Source: CAD feature listing. Evaluate the final solid. Frame: model axes, mm. A direction names the side the tool comes from. Give positions to 0.01 mm unless a question says otherwise; leave off trailing zeros. Loops run counter-clockwise (first coordinate to the right, second up) from the corner with the lowest first, then second, coordinate; pieces in that order, holes last. Notation, with made-up numbers: M -12.75,57 L 0.25,57 A31 cw 0.25,86 Z; hole C 6.25,4.25 d6. An arc over 180 degrees is marked long. Put each result on its own line as item: value.
from build123d import *

# Parameters (mm, degrees)
SKETCH1_W           = 80
SKETCH1_H           = 80
BOSS_EXTRUDE1_DEPTH = 4
CUT_EXTRUDE2_REACH  = 58.71
SKETCH3_R           = 1.75
SKETCH4_W           = 80
SKETCH4_H           = 80
CUT_EXTRUDE3_DEPTH  = 4
SKETCH2_R           = 2.95
BOSS_EXTRUDE2_DEPTH = 8


with BuildPart() as part:
    # Sketch1 → Boss-Extrude1 (new body)
    with BuildSketch(Plane(origin=(0, 0, 0), x_dir=(1, 0, 0), z_dir=(0, 1, 0))):
        Rectangle(SKETCH1_W, SKETCH1_H)
    extrude(amount=BOSS_EXTRUDE1_DEPTH)

    # Sketch3 → Cut-Extrude2 (cut, up to next)
    with BuildSketch(Plane(origin=(0, 4, 0), x_dir=(1, 0, 0), z_dir=(0, 1, 0)), mode=Mode.PRIVATE) as cut_extrude2_sk1:
        with Locations(Location((20.666851305, 33.07387575, 0), (0, 0, 270))):
            Circle(SKETCH3_R)
    cut_extrude2_tool1 = extrude(cut_extrude2_sk1.sketch, amount=-CUT_EXTRUDE2_REACH, mode=Mode.PRIVATE) & part.part
    # Sketch3 → Cut-Extrude2 (cut, up to next)
    with BuildSketch(Plane(origin=(0, 4, 0), x_dir=(1, 0, 0), z_dir=(0, 1, 0)), mode=Mode.PRIVATE) as cut_extrude2_sk2:
        with Locations(Location((-20.666851305, 33.07387575, 0), (0, 0, 90))):
            Circle(SKETCH3_R)
    cut_extrude2_tool2 = extrude(cut_extrude2_sk2.sketch, amount=-CUT_EXTRUDE2_REACH, mode=Mode.PRIVATE) & part.part
    add(cut_extrude2_tool1.solids().sort_by_distance((20.666851, 4, -33.073876))[0], mode=Mode.SUBTRACT)
    add(cut_extrude2_tool2.solids().sort_by_distance((-20.666851, 4, -33.073876))[0], mode=Mode.SUBTRACT)

    # Sketch4 → Cut-Extrude3 (cut)
    with BuildSketch(Plane(origin=(0, 4, 0), x_dir=(1, 0, 0), z_dir=(0, 1, 0))):
        Rectangle(SKETCH4_W, SKETCH4_H)
        Polygon((5, 8), (18.946402637, 37.908156972), (25.290557147, 34.94982914), (6.195338219, -6), (0, -6), (-6.195338219, -6), (-25.290557147, 34.94982914), (-18.946402637, 37.908156972), (-5, 8), (0, 8), align=None, mode=Mode.SUBTRACT)
    extrude(amount=-CUT_EXTRUDE3_DEPTH, mode=Mode.SUBTRACT)

    # Sketch2 → Boss-Extrude2 (add)
    with BuildSketch(Plane(origin=(0, 4, 0), x_dir=(1, 0, 0), z_dir=(0, 1, 0))):
        with Locations(Location((0, 0, 0), (0, 0, 270))):
            Circle(SKETCH2_R)
    extrude(amount=BOSS_EXTRUDE2_DEPTH)


solid = part.part
1. Section query A-A (x = 0). Output: boundary loops of the cut face in (y, z), plus the area to 3 significant figures.
Found:
outline: M 0,-8 L 4,-8 L 4,-2.95 L 12,-2.95 L 12,2.95 L 4,2.95 L 4,6 L 0,6 Z
area: 103 mm^2
2. Draft query along Z for faces 4 (the cylindrical face through (-20.744, 2.028, -31.326)), 5 (the flat face through (11.876, 2.028, -22.745)), 6 (the flat face through (0, 12, 0)). Return one class per face: pulls with the +Z half, pulls with the -Z half, needs draft (parallel to the pull), parting line crosses it, or undercut.
Found:
face 4: undercut
face 5: pulls with the -Z half
face 6: needs draft
3. Material intervals for line 1 (Y direction, x = 5, z = 3.5); line 2 (X direction, y = 3.25, z = -25); line 3 (Z direction, x = 19.5, y = 1.75), sorted ascending. Write a range as from..to.
Found:
line 1: 0..4
line 2: -20.65..-12.93, 12.93..20.65
line 3: -37.65..-34.38, -31.77..-22.53
4. Section query C-C (z = -14). Output: boundary loops of the cut face in (x, y).
Found:
outline: M -15.52,0 L -7.8,0 L -7.8,4 L -15.52,4 Z; M 7.8,0 L 15.52,0 L 15.52,4 L 7.8,4 Z
5. Access query for faces 1 (the cylindrical face through (-2.88, 7.94, -0.64)), 2 (the flat face through (-8, 0, -13)), 3 (the flat face through (0, 2, -8)). Directions: +Z, -Z, +X, -X, +Y, -Y. A direction counts if a zero-diameter tool reaches every point of the face in a straight line with its end or side. Return the directions, or none.
Found:
face 1: +Y
face 2: +Z, -Z, +X, -X, -Y
face 3: -Z, +Y, -Y
6. Contact query for flat-ended pins moving along their axis: P1, Ø4, axis at x = -20.67, z = -33.07, coming from the +Y side; P2, Ø2, axis at x = -1, y = 1.5, coming from the -Z side; P3, Ø5, axis at y = 2, z = -22, coming from the +X side. Output: stop coordinate, or through.
Found:
P1: y = 4
P2: z = -8
P3: x = 20.42
7. Section query D-D (z = 0). Output: boundary loops of the cut face in (x, y), plus the area to 3 significant figures.
Found:
outline: M -8.99,0 L 8.99,0 L 8.99,4 L 2.95,4 L 2.95,12 L -2.95,12 L -2.95,4 L -8.99,4 Z
area: 119 mm^2
8. Section query B-B (y = 3.25). Output: boundary loops of the cut face in (x, z).
Found:
outline: M -25.29,-34.95 L -18.95,-37.91 L -5,-8 L 5,-8 L 18.95,-37.91 L 25.29,-34.95 L 6.2,6 L -6.2,6 Z; hole C -20.67,-33.07 d3.5; hole C 20.67,-33.07 d3.5
